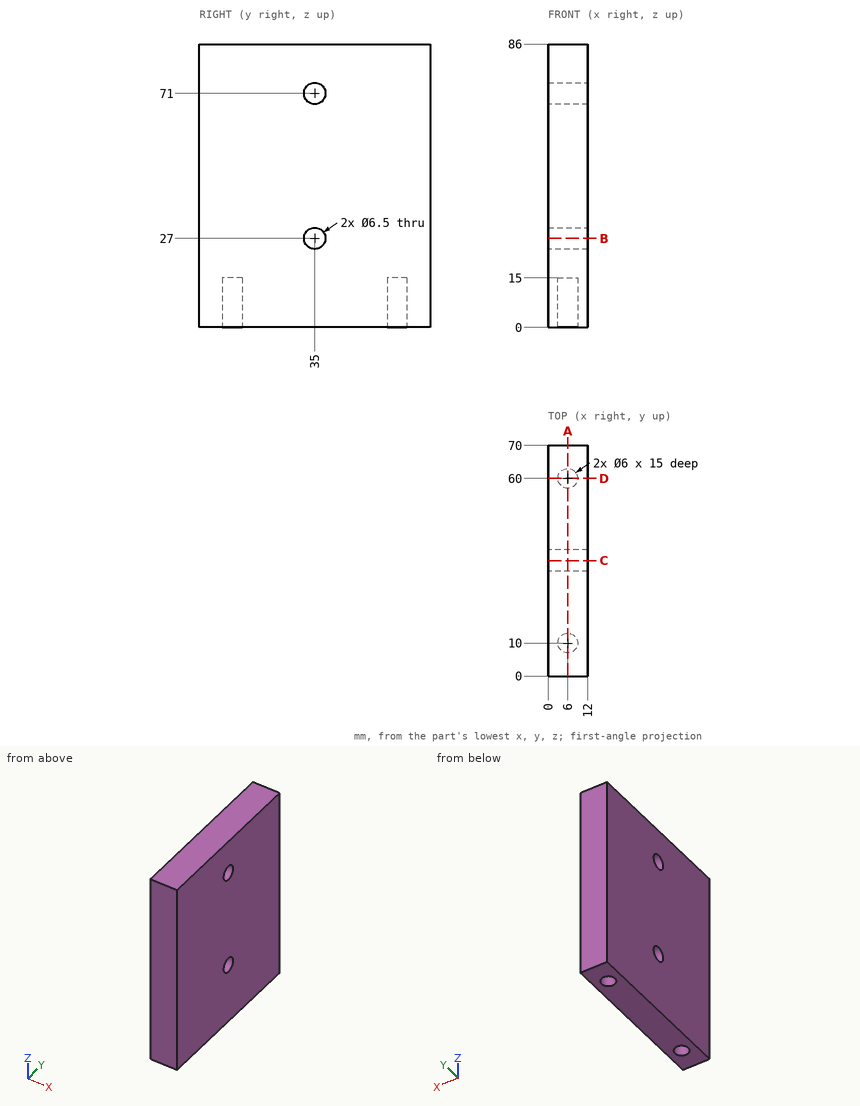
Could you check a few things on this drawing? It's one solid part, dimensions in mm from its lowest x, y, z. Coordinates: 2 decimals unless noted, no trailing zeros. Order: outer loops, then holes, each group sorted by start corner. A loop starts at its lowest first (then second) coordinate and runs counter-clockwise, first axis right, second up.
1) I need wall thicknesses on line 1 (Y direction, x = 6, z = 6.5); line 2 (Y direction, x = 7.25, z = 71); line 3 (Y direction, x = 8.25, z = 6). Which ranges of each line are inside material? Lowest first, please.
2) Imagine slicing it at B-B on z = 27. List the corners of the cut face in (x, y) for me.
3) Imagine slicing it at A-A on x = 6. List the corners of the cut face in (y, z) for me.
4) Imagine slicing it at C-C on y = 35. List the corners of the cut face in (x, z) for me, and give its area (3 significant figures).
5) Imagine slicing it at D-D on y = 60. List the corners of the cut face in (x, z) for me.
6) Will this pin go through, and if not, where does the flat tip stop? pin 1 (5 mm diameter, centred on x = 6, y = 10, fed in from -Z).
Response values:
1. line 1: y = 0 to 7, 13 to 57, 63 to 70
1. line 2: y = 0 to 31.75, 38.25 to 70
1. line 3: y = 0 to 8.02, 11.98 to 58.02, 61.98 to 70
2. outline: (0, 0) - (12, 0) - (12, 31.75) - (0, 31.75) - close; (0, 38.25) - (12, 38.25) - (12, 70) - (0, 70) - close
3. outline: (0, 0) - (7, 0) - (7, 15) - (13, 15) - (13, 0) - (57, 0) - (57, 15) - (63, 15) - (63, 0) - (70, 0) - (70, 86) - (0, 86) - close; hole circle Ø6.5 at (35, 27); hole circle Ø6.5 at (35, 71)
4. outline: (0, 0) - (12, 0) - (12, 23.75) - (0, 23.75) - close; (0, 30.25) - (12, 30.25) - (12, 67.75) - (0, 67.75) - close; (0, 74.25) - (12, 74.25) - (12, 86) - (0, 86) - close
4. area: 876 mm2
5. outline: (0, 0) - (3, 0) - (3, 15) - (9, 15) - (9, 0) - (12, 0) - (12, 86) - (0, 86) - close
6. pin 1: stops at z = 15
